from build123d import *

# Parameters (mm, degrees)
F1_DEPTH = 12.7
F3_DEPTH = 12.7


with BuildPart() as f1:
    # F0 (on Top) → F1 (new body, symmetric)
    with BuildSketch(Plane.XY):
        Polygon((7.88855, 11.681875), (-4.214828, 13.451047), (-13.144354, 5.091305), (-12.175913, -7.102293), (-2.038762, -13.947719), (9.633619, -10.290229), (14.051688, 1.116014), align=None)
    extrude(amount=F1_DEPTH, both=True)

    # F2 (on Right) → F3 (intersect, symmetric)
    with BuildSketch(Plane.YZ):
        Polygon((5.260512, 12.7), (-5.260512, 12.7), (-12.7, 5.260512), (-12.7, -5.260512), (-5.260512, -12.7), (5.260512, -12.7), (12.7, -5.260512), (12.7, 5.260512), align=None)
    extrude(amount=F3_DEPTH, both=True, mode=Mode.INTERSECT)


solid = f1.part
Input: part model. Units: mm. Frame: model coordinates. Round coordinates to 2 decimals unless told otherwise and drop trailing zeros. Order: outer loops, then holes, each group sorted by start corner. A loop starts at its lowest first (then second) coordinate and runs counter-clockwise, first axis right, second up.
1. Pin query (flat end, axial travel): P1, Ø1, axis at x = -9, z = 1.5, coming from the -Y side; P2, Ø1.5, axis at x = -8, y = 5.5, coming from the +Z side; P3, Ø8, axis at x = 9.5, z = -2, coming from the -Y side; P4, Ø10, axis at x = -9.5, z = 7, coming from the -Y side. Return the tip coordinate at first contact, or that it passes through.
The answers:
P1: stops at y = -9.58
P2: stops at z = 12.7
P3: stops at y = -11.59
P4: stops at y = -12.18
2. Mould query, pull axis Z, two halves, no side actions, for faces 1 (the face through (-0.36, 8.1, -9.86)), 2 (the face through (0, 0, 12.7)), 3 (the face through (-12.44, -3.76, 0.18)). Classes: released by +Z, released by -Z, zero draft, split by the parting line, or undercut.
The answers:
face 1: released by -Z
face 2: released by +Z
face 3: zero draft
3. Cut plane D-D, the plane y = 6.75. Output: boundary loops of the cut face in (x, z), then the cut area to 3 significant figures.
The answers:
outline: (-11.37, -11.21) - (10.77, -11.21) - (10.77, 11.21) - (-11.37, 11.21) - close
area: 496 mm2
4. Cut plane C-C, the plane z = 8.75. Output: boundary loops of the cut face in (x, y).
The answers:
outline: (-12.7, -0.5) - (-12.18, -7.1) - (-9.05, -9.21) - (10.05, -9.21) - (12.7, -2.37) - (12.7, 3.43) - (9.33, 9.21) - (-8.74, 9.21) - (-12.7, 5.51) - close
5. Cut plane A-A, the plane z = 3. Output: boundary loops of the cut face in (x, y), then the cut area to 3 significant figures.
The answers:
outline: (-12.7, -0.5) - (-12.18, -7.1) - (-3.89, -12.7) - (1.94, -12.7) - (9.63, -10.29) - (12.7, -2.37) - (12.7, 3.43) - (7.89, 11.68) - (0.92, 12.7) - (-5.02, 12.7) - (-12.7, 5.51) - close
area: 533 mm2
6. Material intervals for line 1 (X direction, y = 8, z = -6); line 2 (Y direction, x = -9.75, z = -11.25); line 3 (Z direction, x = 2.5, y = -6.5), sorted ascending.
The answers:
line 1: x = -10.04 to 10.04
line 2: y = -6.71 to 6.71
line 3: z = -11.46 to 11.46
7. Cut plane B-B, the plane x = 11. Output: boundary loops of the cut face in (y, z), then the cut area to 3 significant figures.
The answers:
outline: (-6.76, -11.2) - (-5.26, -12.7) - (5.26, -12.7) - (6.35, -11.61) - (6.35, 11.61) - (5.26, 12.7) - (-5.26, 12.7) - (-6.76, 11.2) - close
area: 330 mm2
